For this review, use the dimensioned drawing (mm, ordinates from the lowest corner) and the shaded views. A direction names the side the tool comes from. Give positions to 0.01 mm unless a question says otherwise; leave off trailing zeros. Order: outer loops, then holes, each group sorted by start corner. A loop starts at its lowest first (then second) coordinate and runs counter-clockwise, first axis right, second up. Notation, with made-up numbers: M -26,-21.75 L -7,-21.75 A29 cw -7,17.25 Z; hole C 79.5,33.25 d4. An arc over 180 degrees is marked long. Answer as CSV lines item,"result". Start each with the question number.
1. We need section B-B, the plane x = 45. Give the boundary of the cut face in (y, z) (3 decimals), and give its area (3 significant figures).
2. Mouldability with a two-part tool opening along Y and no side actions: class the marked faces 6, 7, 8 and 9 as pulls with the +Y half, pulls with the -Y half, needs draft (parallel to the pull), parting line crosses it, or undercut.
3. We need section D-D, the plane y = 45. Give the boundary of the cut face in (x, z) (3 decimals).
4. We need section A-A, the plane z = 1.5. State how many separate pieces and enclosed holes the cut face has, and give its area (3 significant figures).
5. Machinability: for the marked faces 1, 2, 3, 4 and 5, which of the approach directions +Z, -Z, +X, -X, +Y, -Y give a long, thin tool a straight path to every point of the face, cutting with its end or side? Answer none if there is none.
6. For line 1 along Y through (x, z) = (19, 8); line 2 along Y through (x, z) = (17, 10.25); line 3 along X through (y, z) = (47, 7.75), list the stretches that pass through material, from the lowest coordinate up.
7. Clearance check with flat-ended pins moving along their axes: P1, Ø8, axis at x = 45, y = 59, coming from the -Z side; P2, Ø3.5, axis at x = 62, z = 6, coming from the -Y side; P3, Ø5.5, axis at x = 2.5, z = 4, coming from the +Y side; P4, Ø3.5, axis at y = 58, z = 3, coming from the -X side. State where each tip first meets the part, or that it passes through.
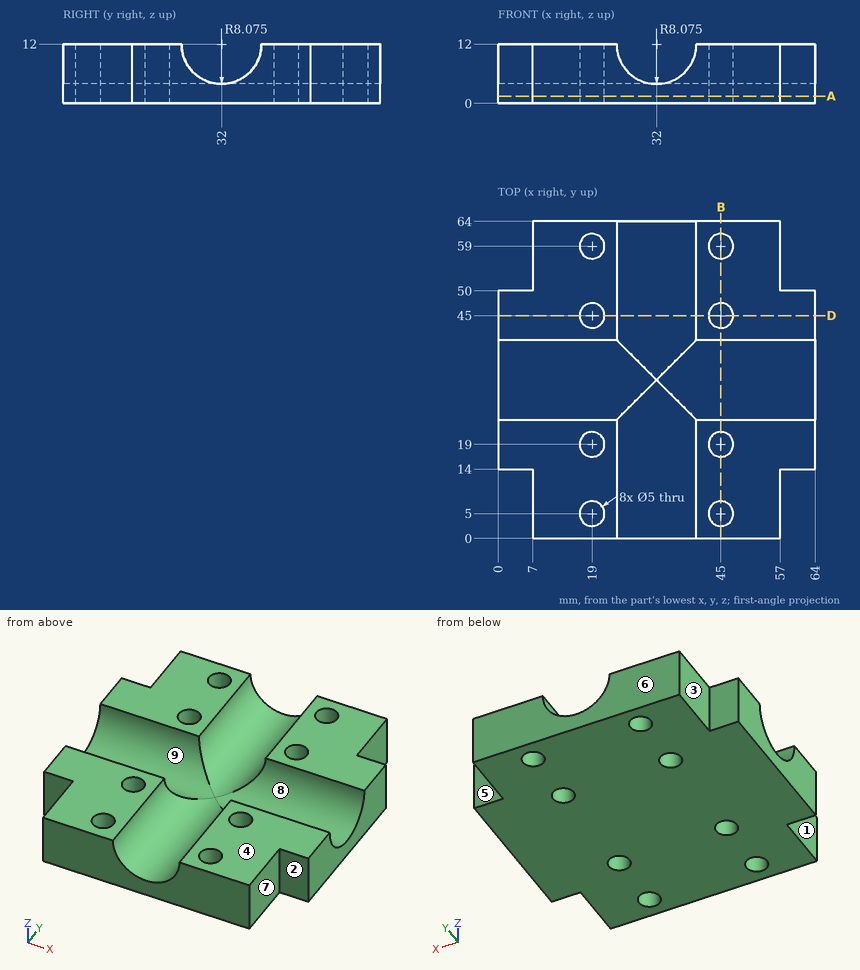
Result set:
1,outline,"M 0,0 L 2.5,0 L 2.5,12 L 0,12 Z; M 7.5,0 L 16.5,0 L 16.5,12 L 7.5,12 Z; M 21.5,0 L 42.5,0 L 42.5,12 L 40.075,12 A8.075 cw 23.925,12 L 21.5,12 Z; M 47.5,0 L 56.5,0 L 56.5,12 L 47.5,12 Z; M 61.5,0 L 64,0 L 64,12 L 61.5,12 Z"
1,area,"426 mm2"
2,face 6,"pulls with the +Y half"
2,face 7,"needs draft"
2,face 8,"undercut"
2,face 9,"undercut"
3,outline,"M 0,0 L 16.5,0 L 16.5,12 L 0,12 Z; M 21.5,0 L 42.5,0 L 42.5,12 L 40.075,12 A8.075 cw 23.925,12 L 21.5,12 Z; M 47.5,0 L 64,0 L 64,12 L 47.5,12 Z"
4,separate pieces,"1"
4,enclosed holes,"8"
4,area,"3,550 mm2"
5,face 1,"+Z, -Z, -X, -Y"
5,face 2,"+Z, -Z, +X, -Y"
5,face 3,"+Z, -Z, -X, +Y"
5,face 4,"+Z, +X, -X, +Y, -Y"
5,face 5,"+Z, -Z, +X, +Y"
6,line 1,"0 to 2.5, 7.5 to 16.5, 21.5 to 24.99, 39.01 to 42.5, 47.5 to 56.5, 61.5 to 64"
6,line 2,"0 to 3.5, 6.5 to 17.5, 20.5 to 24.12, 39.88 to 43.5, 46.5 to 57.5, 60.5 to 64"
6,line 3,"0 to 17.5, 20.5 to 25.13, 38.87 to 43.5, 46.5 to 64"
7,P1,"z = 0"
7,P2,"y = 14"
7,P3,"y = 50"
7,P4,"x = 7"
